Could you check a few things on this model? Use its own coordinates, in mm. Face numbers are marked on the shaded views. A direction names the side the tool comes from. Coordinates: 2 decimals unless noted, no trailing zeros. Loops run counter-clockwise (first coordinate to the right, second up) from the corner with the lowest first, then second, coordinate; pieces in that order, holes last.
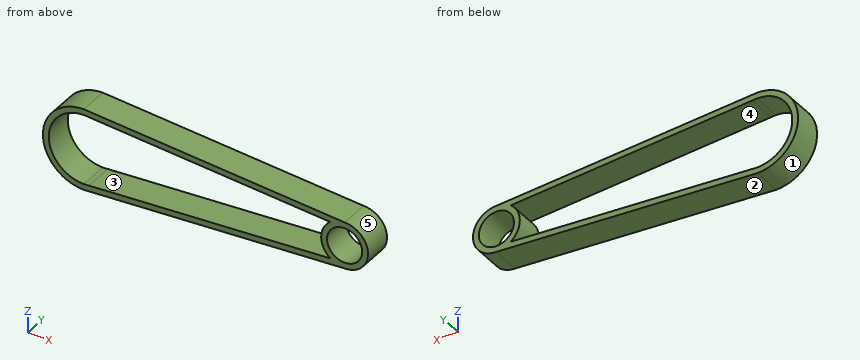
from build123d import *

# Parameters (mm, degrees)
SKETCH1_R           = 6
BOSS_EXTRUDE1_DEPTH = 10


with BuildPart() as part:
    # Sketch1 → Boss-Extrude1 (new body)
    with BuildSketch(Plane(origin=(0, 0, 0), x_dir=(1, 0, 0), z_dir=(0, 1, 0))):
        with BuildLine():
            ThreePointArc((0, 14), (-14, 0), (0, -14))
            Line((0, -14), (89, -8))
            ThreePointArc((89, -8), (97, 0), (89, 8))
            Line((89, 8), (0, 14))
        make_face()
        with BuildLine():
            ThreePointArc((1.674796148, -11.882552666), (0.807156628, -11.972823317), (-0.064748194, -11.999825318))
            ThreePointArc((-0.064748194, -11.999825318), (-12, 0), (-0.064748194, 11.999825318))
            ThreePointArc((-0.064748194, 11.999825318), (0.807156628, 11.972823317), (1.674796148, 11.882552666))
            Line((1.674796148, 11.882552666), (84.102414172, 6.325634597))
            ThreePointArc((84.102414172, 6.325634597), (81, 0), (84.102414172, -6.325634597))
            Line((84.102414172, -6.325634597), (1.674796148, -11.882552666))
        make_face(mode=Mode.SUBTRACT)
        with Locations((89, 0)):
            Circle(SKETCH1_R, mode=Mode.SUBTRACT)
    extrude(amount=BOSS_EXTRUDE1_DEPTH)


solid = part.part
(1) We'd pull the mould along Z, two halves only. Please class the marked faces 1, 2 and 3: +Z half, -Z half, draft (parallel to the pull), parting line (faces both ways), or undercut.
Answers:
face 1: parting line
face 2: -Z half
face 3: undercut
(2) Imagine slicing it at C-C, the plane x = 63.5. Write out the boundary of the cut face in (y, z).
Answers:
outline: (0, -9.72) - (10, -9.72) - (10, -7.71) - (0, -7.71) - close; (0, 7.71) - (10, 7.71) - (10, 9.72) - (0, 9.72) - close
(3) I need wall thicknesses on probe 1 along X at (y, z) = (5.75, 0); probe 2 along Z at (x, y) = (89, 2.5); probe 3 along Z at (x, y) = (48, 4.5). Which ranges of each line are inside material? Lowest first, please.
Answers:
probe 1: x = -14 to -12, 81 to 83, 95 to 97
probe 2: z = -8 to -6, 6 to 8
probe 3: z = -10.76 to -8.76, 8.76 to 10.76
(4) Imagine slicing it at B-B, the plane y = 2.75. Write out the boundary of the cut face in (x, z), and give its area (3 significant figures).
Answers:
outline: (0, -14) - (89, -8) arc R8 ccw to (89, 8) - (0, 14) arc R14 ccw to start; hole (1.67, -11.88) - (84.1, -6.33) arc R8 cw to (84.1, 6.33) - (1.67, 11.88) arc R12 ccw (long way) to start; hole circle Ø12 at (89, 0)
area: 514 mm2
(5) Imagine slicing it at A-A, the plane z = 0. Write out the boundary of the cut face in (x, y), and give its area (3 significant figures).
Answers:
outline: (-14, 0) - (-12, 0) - (-12, 10) - (-14, 10) - close; (81, 0) - (83, 0) - (83, 10) - (81, 10) - close; (95, 0) - (97, 0) - (97, 10) - (95, 10) - close
area: 60.0 mm2
(6) For pin 1 (2 mm diameter, centred on y = 8.5, z = -0.5, fed in from -X); pin 2 (6 mm diameter, centred on x = 23.5, y = 8, fed in from -Z); pin 3 (1.5 mm diameter, centred on x = 82, y = 2, fed in from +Z); pin 4 (5 mm diameter, centred on y = 5.5, z = 7.5, fed in from +X) (3 decimals), each with a flat end and sliding along its axis, tell me the tip position at first contact or that it passes through.
Answers:
pin 1: stops at x = -14
pin 2: stops at z = -12.62
pin 3: stops at z = 8.52
pin 4: stops at x = 95.245
(7) Which directions (+Z, -Z, +X, -X, +Y, -Y) give clear straight access to the entire face, cutting with the end or side of a thin tool? Please do the marked faces 4 and 5.
Answers:
face 4: +Y, -Y
face 5: +X, +Y, -Y
